Verification items for the finished model (mm, model axes). Face numbers are marked on the shaded views. A direction names the side the tool comes from. Coordinates: 2 decimals unless noted, no trailing zeros. Order: outer loops, then holes, each group sorted by start corner. A loop starts at its lowest first (then second) coordinate and runs counter-clockwise, first axis right, second up. Notation, with made-up numbers: (31.5, -5.5) -> (37.5, -5.5) arc R17 ccw to (37.5, 11.5) -> close; hole circle Ø6 at (38.5, -40). An arc over 180 degrees is marked (long way). Answer as CSV lines item,"result".
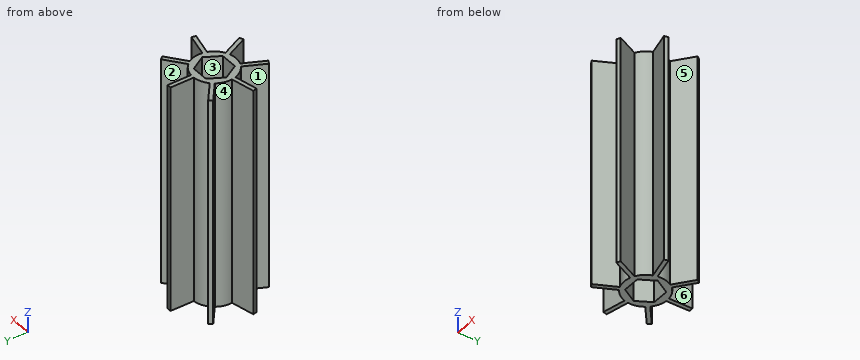
```python
from build123d import *

# Parameters (mm, degrees)
BOSS_EXTRUDE1_DEPTH = 76.2
SKETCH6_R           = 7.239
BOSS_EXTRUDE2_DEPTH = 76.2
CIRPATTERN1_COUNT   = 7
CUT_EXTRUDE5_DEPTH  = 80.057508243


with BuildPart() as part:
    # Sketch12 → Boss-Extrude1 (new body)
    with BuildSketch(Plane.XY):
        Polygon((0, 0), (0.8406384, 0), (0.8406384, 14.987843642), (-0.5309616, 14.987843642), (-0.5309616, 0), align=None)
    boss_extrude1 = extrude(amount=-BOSS_EXTRUDE1_DEPTH)

    # Sketch6 → Boss-Extrude2 (add)
    with BuildSketch(Plane.XY):
        Circle(SKETCH6_R)
    extrude(amount=-BOSS_EXTRUDE2_DEPTH)

    # CirPattern1: Boss-Extrude1 ×7 about axis
    cirpattern1_axis = Axis((0, 0, 0), (0, 0, 1))
    for i in range(1, CIRPATTERN1_COUNT):
        add(boss_extrude1.rotate(cirpattern1_axis, i * 360 / CIRPATTERN1_COUNT))

    # Sketch8 → Cut-Extrude5 (cut, through all)
    with BuildSketch(Plane.XY):
        Polygon((5.6310401, 0.047871874), (2.774061791, 4.900559713), (-2.856978309, 4.852687839), (-5.6310401, -0.047871874), (-2.774061791, -4.900559713), (2.856978309, -4.852687839), align=None)
    extrude(amount=-CUT_EXTRUDE5_DEPTH, mode=Mode.SUBTRACT)


solid = part.part
```
Item 1: Section check C-C, the plane y = -8.75. Record the boundary of the cut face in (x, z), plus the area to 3 significant figures.
Answer list:
outline,"(-5.15, -76.2) -> (-3.62, -76.2) -> (-3.62, 0) -> (-5.15, 0) -> close; (3.28, -76.2) -> (4.8, -76.2) -> (4.8, 0) -> (3.28, 0) -> close"
area,"232 mm2"
Item 2: Release check for a two-part mould opening along X. For the marked faces 4, 5 and 6 record: +X half, -X half, draft (parallel to the pull), parting line (faces both ways), or undercut.
Answer list:
face 4,"-X half"
face 5,"+X half"
face 6,"undercut"
Item 3: Depth check by flat-ended pin: pin 1 Ø8.5 at (y, z) = (10, -23) entering from -X; pin 2 Ø2.5 at (y, z) = (11.5, -27) entering from +X; pin 3 Ø2 at (x, z) = (3.5, -18.5) entering from -Y; pin 4 Ø4 at (x, y) = (2, 1.5) entering from +Z. Enter the tip coordinate at first touch or a pass-through.
Answer list:
pin 1,"x = -12.05"
pin 2,"x = 0.84"
pin 3,"y = -11.28"
pin 4,"through"
Item 4: Thickness scan on line 1 (X direction, y = 7.75, z = -48); line 2 (Y direction, x = -4, z = -12); line 3 (X direction, y = 8.75, z = -36.5). Record the ranges inside material, lowest first.
Answer list:
line 1,"-10.57 to -8.37, -0.53 to 0.84, 8.87 to 11.07"
line 2,"-9.53 to -6.37, -6.03 to -2.82, 2.83 to 6.03"
line 3,"-11.82 to -9.62, -0.53 to 0.84, 10.12 to 12.19"
Item 5: Section check A-A, the plane x = -8. Record the boundary of the cut face in (y, z) (3 decimals).
Answer list:
outline,"(-2.371, -76.2) -> (-0.964, -76.2) -> (-0.964, 0) -> (-2.371, 0) -> close; (5.701, -76.2) -> (7.455, -76.2) -> (7.455, 0) -> (5.701, 0) -> close"
Item 6: Section check D-D, the plane y = 13.25. Record the boundary of the cut face in (x, z).
Answer list:
outline,"(-0.53, -76.2) -> (0.84, -76.2) -> (0.84, 0) -> (-0.53, 0) -> close"
Item 7: Tool access check on the marked faces 1, 2 and 3. Record the directions out of +Z, -Z, +X, -X, +Y, -Y that give a thin tool (end or side, any length) a straight path to the whole face; none if there is none.
Answer list:
face 1,"+Z, -Z, -X"
face 2,"+Z, -Z, +Y"
face 3,"+Z, -Z"
